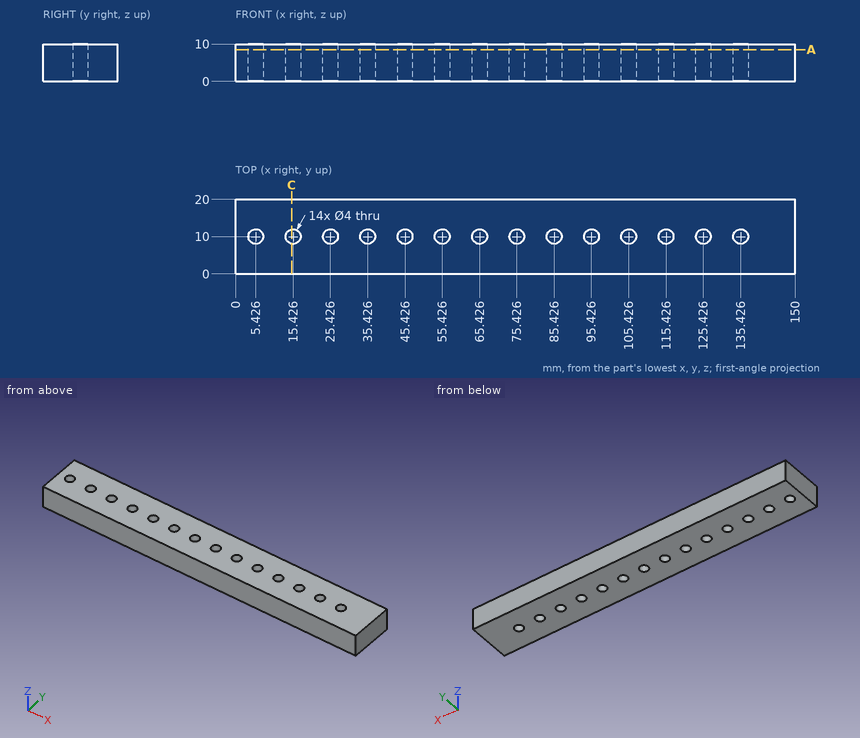
Print and shaded views of the part. All mm, measured from the part's lowest x, y and z. Give positions to 0.01 mm unless a question says otherwise; leave off trailing zeros. Loops run counter-clockwise (first coordinate to the right, second up) from the corner with the lowest first, then second, coordinate; pieces in that order, holes last. Notation, with made-up numbers: (48, -16) - (92, -16) arc R10 cw to (92, -3) - close; hole circle Ø8 at (-31.5, 58). An arc over 180 degrees is marked (long way). One line per item, written item: value. Start each with the question number.
1. Pin check, flat tip, straight feed: pin 1 (2.5 mm diameter, centred on x = 15.43, y = 10, fed in from +Z). Stop position of the tip, or through.
2. Slice it at A-A (z = 8.5). Give the number of separate pieces and of enclosed holes in the cut face, plus the area to 3 significant figures.
3. Probe L1, parallel to Y at x = 35.5, z = 1; L2, parallel to Y at x = 37, z = 1.75. List the from-to ranges inside material, lowest first. Write a range as from..to.
4. Slice it at C-C (x = 15). List the corners of the cut face in (y, z).
Solution:
1. pin 1: passes through
2. separate pieces: 1
2. enclosed holes: 14
2. area: 2,820 mm^2
3. L1: y = 0..8, 12..20
3. L2: y = 0..8.77, 11.23..20
4. outline: (0, 0) - (8.05, 0) - (8.05, 10) - (0, 10) - close; (11.95, 0) - (20, 0) - (20, 10) - (11.95, 10) - close
